from build123d import *

# Parameters (mm, degrees)
SKETCH1_W           = 20
SKETCH1_H           = 540
BOSS_EXTRUDE1_DEPTH = 150
SKETCH2_W           = 540
SKETCH2_H           = 20
BOSS_EXTRUDE2_DEPTH = 36
M10_TAPPED_HOLE1_D  = 8.5


with BuildPart() as part:
    # Sketch1 → Boss-Extrude1 (new body)
    with BuildSketch(Plane(origin=(0, 0, 0), x_dir=(1, 0, 0), z_dir=(0, 1, 0))):
        with Locations((10, 0)):
            Rectangle(SKETCH1_W, SKETCH1_H)
    extrude(amount=BOSS_EXTRUDE1_DEPTH)

    # Sketch2 → Boss-Extrude2 (add)
    with BuildSketch(Plane(origin=(0, 0, 0), x_dir=(0, 0, -1), z_dir=(1, 0, 0))):
        with Locations((0, 10)):
            Rectangle(SKETCH2_W, SKETCH2_H)
    extrude(amount=-BOSS_EXTRUDE2_DEPTH)

    # M10 Tapped Hole1 (through all)
    with Locations(Plane(origin=(-16, 150, -240), x_dir=(0, 0, 1), z_dir=(0, 1, 0))):
        with Locations((0, 0), (80, 0), (160, 0)):
            m10_tapped_hole1 = Hole(M10_TAPPED_HOLE1_D / 2)

    # Mirror1: M10 Tapped Hole1 across plane
    add(m10_tapped_hole1.mirror(Plane.XY), mode=Mode.SUBTRACT)


solid = part.part
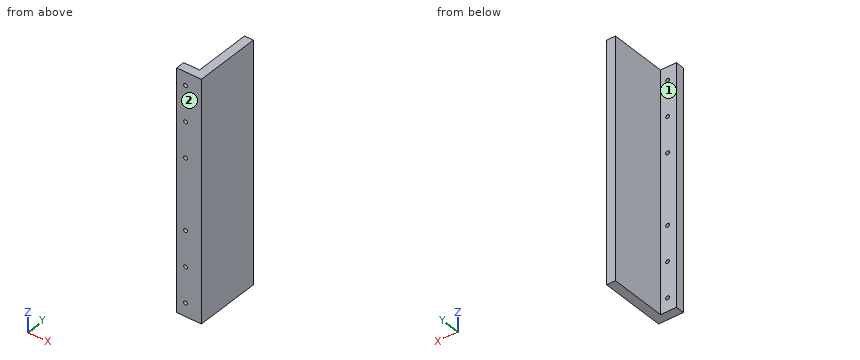
Geometry check sheet. Reference: the model listing, model coordinates, mm. Face numbers are marked on the shaded views. A direction names the side the tool comes from. Coordinates: 2 decimals unless noted, no trailing zeros. Order: outer loops, then holes, each group sorted by start corner. A loop starts at its lowest first (then second) coordinate and runs counter-clockwise, first axis right, second up. Notation, with made-up numbers: (28.25, 58) - (79.25, 58) arc R29 ccw to (79.25, 82) - close; hole circle Ø6 at (-23.75, 86). An arc over 180 degrees is marked (long way). Answer in a Markdown table with one row per item. Add a question column.
1) Cross-section at B-B, the plane y = 33. Record the cut outline in (x, z), then the cut area to 3 significant figures.
2) Gauge pin test, flat ends, axial feed: P1, Ø10, axis at x = -25.5, z = -11.5, coming from the -Y side; P2, Ø5, axis at x = -16, z = -80, coming from the -Y side; P3, Ø5, axis at y = 125.5, z = -185.5, coming from the -X side; P4, Ø11, axis at x = -16, z = 160, coming from the +Y side. Record the tip position at first contact, or that the pin passes through.
3) Set-up check for the marked faces 1 and 2: record each of +Z, -Z, +X, -X, +Y, -Y from which the full face is reachable in a straight line by a thin tool's end or side.
4) Cross-section at A-A, the plane z = -202.5. Record the cut outline in (x, y), then the cut area to 3 significant figures.
5) Material ranges on line 1 along X through (y, z) = (5, 80); line 2 along X through (y, z) = (55, -159), recorded low to high. Write a range as [from, to].
Check result:
| question | item | result |
|---|---|---|
| 1 | outline | (0, -270) - (20, -270) - (20, 270) - (0, 270) - close |
| 1 | area | 10,800 mm² |
| 2 | P1 | stops at y = 0 |
| 2 | P2 | passes through |
| 2 | P3 | stops at x = 0 |
| 2 | P4 | stops at y = 20 |
| 3 | face 1 | +Z, -Z, -X, +Y |
| 3 | face 2 | +Z, -Z, +X, -X, -Y |
| 4 | outline | (-36, 0) - (20, 0) - (20, 150) - (0, 150) - (0, 20) - (-36, 20) - close |
| 4 | area | 3,720 mm² |
| 5 | line 1 | x = [-36, -20.25], [-11.75, 20] |
| 5 | line 2 | x = [0, 20] |
